Can you work these out from the model? Positions are in its coordinate system, mm. Face numbers are marked on the shaded views. Give positions to 0.01 mm unless a question says otherwise; leave off trailing zeros. Loops run counter-clockwise (first coordinate to the right, second up) from the corner with the lowest first, then second, coordinate; pieces in that order, holes last. Notation, with made-up numbers: M -2.5,63.5 L 41.5,63.5 A34 cw 41.5,93.5 Z; hole C 77,56 d5. An arc over 180 degrees is marked long. Put each result on its own line as item: value. Start each with the question number.
1) Please list where these lines run through material, in increasing order: line 1 along X through (y, z) = (1.3, -7.5); line 2 along X through (y, z) = (1.45, -25.5); line 3 along Z through (x, y) = (-27, 2). Write a range as from..to.
2) Imagine slicing it at D-D (z = -41.5). Write out the boundary of the cut face in (x, y), then the cut area to 4 significant figures.
3) Imagine slicing it at C-C (y = 5.25). Write out the boundary of the cut face in (x, z), then the cut area to 3 significant figures.
4) If we mould it in two halves opening along X, with no side actions, what happens to the marked faces 1 and 2? For each: +X half, -X half, draft (parallel to the pull), parting line (faces both ways), or undercut.
5) Imagine slicing it at B-B (z = -25.5). Write out the boundary of the cut face in (x, y), then the cut area to 4 significant figures.
6) For P1, Ø1.5, axis at x = -36.5, z = -29.5, coming from the +Y side; P2, Ø4, axis at x = -39, z = -25.5, coming from the +Y side; P3, Ø3, axis at x = -34.5, z = -8, coming from the -Y side, each with a flat end and sliding along its axis, tell me the tip position at first contact or that it passes through.
7) Imagine slicing it at A-A (x = -5). Write out the boundary of the cut face in (y, z).
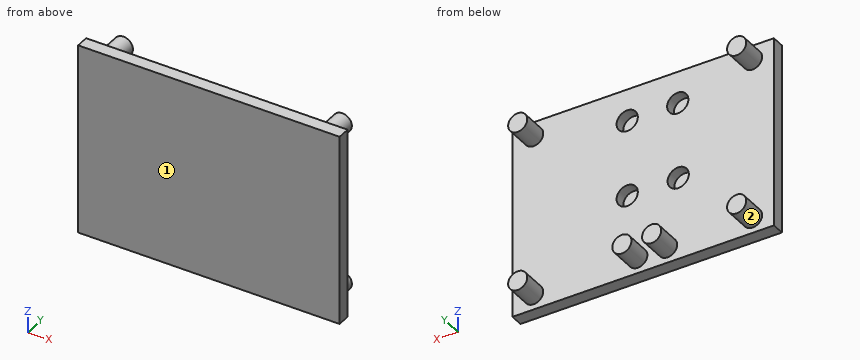
Autodesk Inventor part; units mm, degrees
ref_plane "YZ Plane" through (0, 0, 0) normal (1, 0, 0) x (0, 1, 0)
ref_plane "XZ Plane" through (0, 0, 0) normal (0, 1, 0) x (-1, 0, 0)
ref_plane "XY Plane" through (0, 0, 0) normal (0, 0, 1) x (1, 0, 0)
sketch "Sketch1" plane through (0, 0, 0) normal (0, 1, 0) x (-1, 0, 0)
  line L0 (0, 0) -> (61.5, 0)
  line L1 (61.5, 0) -> (61.5, -45)
  line L2 (61.5, -45) -> (0, -45)
  line L3 (0, -45) -> (0, 0)
  dimension "d0" = 61.5
  dimension "d1" = 45
extrude "Extrusion1" add sketch "Sketch1" along normal blind 3
sketch "Sketch2" plane through (0, 3, 0) normal (0, 1, 0) x (1, 0, 0)
  circle A0 centre (-27, 25.5) radius 2.5
  line L0 (0, 0) -> (0, 45)
  line L1 (-61.5, 0) -> (0, 0)
  line L2 (0, 45) -> (-61.5, 45)
  circle A1 centre (-39, 25.4996) radius 2.5
  circle A2 centre (-38.887, 7.5) radius 2.5
  circle A3 centre (-27, 7.5) radius 2.5
  dimension "d4" = 5
  dimension "d5" = 27
  dimension "d8" = 5
  dimension "d9" = 12
  dimension "d10" = 5
  dimension "d11" = 18
  dimension "d12" = 5
  dimension "d13" = 7.5
  dimension "d14" = 7.5
  dimension "d15" = 18
hole "Hole1" at (-27, 3, -7.5) at (-38.887, 3, -7.5) at (-39, 3, -25.4996) at (-27, 3, -25.5) direction (0, -1, 0) diameter 5 depth 2.5
sketch "Sketch3" plane through (0, 3, 0) normal (0, 1, 0) x (1, 0, 0)
  circle A0 centre (-5, 3.5) radius 2.25
  line L0 (-61.5, 0) -> (0, 0)
  line L1 (0, 0) -> (0, 45)
  circle A1 centre (-56.5, 3.5) radius 2.25
  line L2 (-61.5, 45) -> (-61.5, 0)
  circle A2 centre (-5, 41.5) radius 2.25
  line L3 (0, 45) -> (-61.5, 45)
  circle A3 centre (-56.5, 41.5) radius 2.25
  circle A4 centre (-29.5, 41.5) radius 2.25
  circle A5 centre (-36.5, 41.5) radius 2.25
  dimension "d23" = 4.5
  dimension "d24" = 3.5
  dimension "d25" = 5
  dimension "d26" = 4.5
  dimension "d27" = 3.5
  dimension "d28" = 5
  dimension "d29" = 4.5
  dimension "d30" = 3.5
  dimension "d31" = 4.5
  dimension "d32" = 4.5
  dimension "d33" = 24.5
  dimension "d34" = 5
  dimension "d35" = 5
  dimension "d36" = 3.5
  dimension "d37" = 4.5
  dimension "d38" = 20
extrude "Extrusion2" add sketch "Sketch3" along normal blind 6 contours A0 | A1 | A2 | A3 | A4 | A5
properties part number "TrolleyTopPlate1"
Recorded:
1. line 1: -61.5..-41.39, -36.39..-29.5, -24.5..0
1. line 2: -61.5..-41.5, -36.5..-29.5, -24.5..0
1. line 3: -45..-28, -23..-10, -5..0
2. outline: M -61.5,0 L 0,0 L 0,3 L -2.75,3 L -2.75,9 L -7.25,9 L -7.25,3 L -27.25,3 L -27.25,9 L -31.75,9 L -31.75,3 L -34.25,3 L -34.25,9 L -38.75,9 L -38.75,3 L -54.25,3 L -54.25,9 L -58.75,9 L -58.75,3 L -61.5,3 Z
2. area: 292.5 mm²
3. outline: C -56.5,-41.5 d4.5; C -56.5,-3.5 d4.5; C -36.5,-41.5 d4.5; C -29.5,-41.5 d4.5; C -5,-41.5 d4.5; C -5,-3.5 d4.5
3. area: 95.4 mm²
4. face 1: draft
4. face 2: undercut
5. outline: M -61.5,0 L 0,0 L 0,3 L -24.5,3 L -24.5,0.5 L -29.5,0.5 L -29.5,3 L -36.5,3 L -36.5,0.5 L -41.5,0.5 L -41.5,3 L -61.5,3 Z
5. area: 159.5 mm²
6. P1: y = 3
6. P2: y = 0.5
6. P3: y = 0
7. outline: M 0,-45 L 3,-45 L 3,-43.75 L 9,-43.75 L 9,-39.25 L 3,-39.25 L 3,-5.75 L 9,-5.75 L 9,-1.25 L 3,-1.25 L 3,0 L 0,0 Z
